Check sheet for the modelled part. Datum: model origin and axes. Units: mm. A direction names the side the tool comes from. Give positions to 0.01 mm unless a question says otherwise; leave off trailing zeros. Loops run counter-clockwise (first coordinate to the right, second up) from the corner with the lowest first, then second, coordinate; pieces in that order, holes last. Notation, with made-up numbers: (1, 22.5) - (22, 22.5) arc R29 cw to (22, 54.5) - close; hole circle Ø9 at (83.25, 6). An arc over 180 degrees is marked (long way). Use one line per item in the form item = value.
from build123d import *

# Parameters (mm, degrees)
SKETCH_1_R      = 2.5
SKETCH_1_R_2    = 1.75
SKETCH_1_W      = 13
SKETCH_1_H      = 24
EXTRUDE_1_DEPTH = 5


with BuildPart() as part:
    # 스케치1 → 보스-돌출1 (new body)
    with BuildSketch(Plane.XY):
        with BuildLine():
            Line((-85.42, 22.575), (85.42, 22.575))
            ThreePointArc((85.42, 22.575), (88.92, 19.075), (85.42, 15.575))
            Line((85.42, 15.575), (14.5, 15.575))
            Line((14.5, 15.575), (14.5, -22.575))
            ThreePointArc((14.5, -22.575), (0, -37.075), (-14.5, -22.575))
            Line((-14.5, -22.575), (-14.5, 15.575))
            Line((-14.5, 15.575), (-85.42, 15.575))
            ThreePointArc((-85.42, 15.575), (-88.92, 19.075), (-85.42, 22.575))
        make_face()
        with Locations((-85.42, 19.075)):
            Circle(SKETCH_1_R, mode=Mode.SUBTRACT)
        with Locations((85.42, 19.075)):
            Circle(SKETCH_1_R, mode=Mode.SUBTRACT)
        with Locations((-11.199423754, -25.875576246)):
            Circle(SKETCH_1_R_2, mode=Mode.SUBTRACT)
        with Locations((11.199423754, -25.875576246)):
            Circle(SKETCH_1_R_2, mode=Mode.SUBTRACT)
        with Locations((0, -2.676152492)):
            Rectangle(SKETCH_1_W, SKETCH_1_H, mode=Mode.SUBTRACT)
    extrude(amount=EXTRUDE_1_DEPTH)


solid = part.part
Item 1: Gauge pin test, flat ends, axial feed: P1, Ø2, axis at x = 66.5, z = 0.5, coming from the -Y side (3 decimals); P2, Ø5.5, axis at x = -11.2, y = -25.88, coming from the -Z side; P3, Ø4, axis at x = -85.42, y = 19.075, coming from the -Z side; P4, Ø2.5, axis at y = -5, z = 3, coming from the -X side. Record the tip position at first contact, or that the pin passes through.
Answer block:
P1 = 15.575
P2 = 0
P3 = through
P4 = -14.5
Item 2: Section check B-B on z = 1.1. Record the boundary of the cut face in (x, y) (3 decimals).
Answer block:
outline = (-85.42, 15.575) - (-14.5, 15.575) - (-14.5, -22.575) arc R14.5 ccw to (14.5, -22.575) - (14.5, 15.575) - (85.42, 15.575) arc R3.5 ccw to (85.42, 22.575) - (-85.42, 22.575) arc R3.5 ccw to start; hole circle Ø5 at (-85.42, 19.075); hole circle Ø3.5 at (-11.199, -25.876); hole (-6.5, -14.676) - (6.5, -14.676) - (6.5, 9.324) - (-6.5, 9.324) - close; hole circle Ø3.5 at (11.199, -25.876); hole circle Ø5 at (85.42, 19.075)
Item 3: Section check C-C on x = 68. Record the boundary of the cut face in (y, z) (3 decimals).
Answer block:
outline = (15.575, 0) - (22.575, 0) - (22.575, 5) - (15.575, 5) - close
Item 4: Section check A-A on x = 0. Record the boundary of the cut face in (y, z) (3 decimals).
Answer block:
outline = (-37.075, 0) - (-14.676, 0) - (-14.676, 5) - (-37.075, 5) - close; (9.324, 0) - (22.575, 0) - (22.575, 5) - (9.324, 5) - close
Item 5: Thickness scan on L1, parallel to X at y = -14, z = 3.25; L2, parallel to Y at x = 85.42, z = 3.75 (3 decimals); L3, parallel to Y at x = -41, z = 3.2 (3 decimals). Record the ranges inside material, lowest first.
Answer block:
L1 = -14.5 to -6.5, 6.5 to 14.5
L2 = 15.575 to 16.575, 21.575 to 22.575
L3 = 15.575 to 22.575
Item 6: Mould release check, pull along X, two halves, no side actions. Record for faces 1 (the face through (88.92, 19.15, 2.46)), 2 (the face through (0, 9.324, 2)), 3 (the face through (7, 2, 5)), 4 (the face through (6.5, -3, 2)): released by +X, released by -X, zero draft, split by the parting line, or undercut.
Answer block:
face_1 = released by +X
face_2 = undercut
face_3 = zero draft
face_4 = undercut
Item 7: Access from +Z, -Z, +X, -X, +Y, -Y to the whole of each face (thin tool, end or side, straight path). Record for faces 5 (the face through (14.5, -3, 2)), 6 (the face through (0, -14.676, 2)), 7 (the face through (-1, 22.575, 2)), 8 (the face through (7, 2, 0)), 9 (the face through (-49, 15.575, 2)).
Answer block:
face_5 = +Z, -Z, +X, -Y
face_6 = +Z, -Z
face_7 = +Z, -Z, +X, -X, +Y
face_8 = -Z, +X, -X, +Y, -Y
face_9 = +Z, -Z, -X, -Y
